```python
from build123d import *

# Parameters (mm, degrees)
SKETCH1_W           = 290
SKETCH1_H           = 154.65
BOSS_EXTRUDE1_DEPTH = 3
SKETCH2_W           = 21
SKETCH2_H           = 40.5
CUT_EXTRUDE1_DEPTH  = 165.356793669
CUT_EXTRUDE2_DEPTH  = 165.356793669
SKETCH4_W           = 24
SKETCH4_H           = 10.25
BOSS_EXTRUDE2_DEPTH = 3


with BuildPart() as part:
    # Sketch1 → Boss-Extrude1 (new body)
    with BuildSketch(Plane(origin=(0, 0, 0), x_dir=(1, 0, 0), z_dir=(0, 1, 0))):
        Rectangle(SKETCH1_W, SKETCH1_H)
    extrude(amount=BOSS_EXTRUDE1_DEPTH)

    # Sketch2 → Cut-Extrude1 (cut, through all)
    with BuildSketch(Plane(origin=(0, 3, 0), x_dir=(1, 0, 0), z_dir=(0, 1, 0))):
        with Locations((0, 57.075)):
            Rectangle(SKETCH2_W, SKETCH2_H)
    extrude(amount=-CUT_EXTRUDE1_DEPTH, mode=Mode.SUBTRACT)

    # Sketch3 → Cut-Extrude2 (cut, through all)
    with BuildSketch(Plane(origin=(0, 3, 0), x_dir=(1, 0, 0), z_dir=(0, 1, 0))):
        Polygon((-116, -73.825), (-116, -77.325), (-88.5, -77.325), (-88.5, -66.325), (-112, -66.325), (-112, -61.825), (-124, -61.825), (-124, -73.825), align=None)
    extrude(amount=-CUT_EXTRUDE2_DEPTH, mode=Mode.SUBTRACT)

    # Sketch4 → Boss-Extrude2 (add, through all)
    with BuildSketch(Plane(origin=(0, 3, 0), x_dir=(1, 0, 0), z_dir=(0, 1, 0))):
        with Locations((-133, -82.45)):
            Rectangle(SKETCH4_W, SKETCH4_H)
    extrude(amount=-BOSS_EXTRUDE2_DEPTH)


solid = part.part
```
Check sheet for the modelled part. Datum: model origin and axes. Units: mm. Coordinates: 2 decimals unless noted, no trailing zeros. Loops run counter-clockwise (first coordinate to the right, second up) from the corner with the lowest first, then second, coordinate; pieces in that order, holes last.
1) Gauge pin test, flat ends, axial feed: pin 1 (4 mm diameter, centred on x = 49, z = 11.5, fed in from -Y); pin 2 (0.9 mm diameter, centred on x = -103.5, y = 1, fed in from +Z) (3 decimals); pin 3 (1.5 mm diameter, centred on x = 62.5, y = 1, fed in from +Z) (3 decimals). Record the tip position at first contact, or that the pin passes through.
2) Material ranges on probe 1 along X at (y, z) = (1.4, 64.5); probe 2 along X at (y, z) = (2.5, -48.5); probe 3 along Z at (x, y) = (-11, 2.4) (3 decimals), recorded low to high.
3) Sectioned sample at D-D (x = 123). Record the boundary of the cut face in (y, z) (3 decimals).
4) Sectioned sample at B-B (y = 1.5). Record the boundary of the cut face in (x, z) (3 decimals).
5) Sectioned sample at C-C (x = -7). Record the boundary of the cut face in (y, z) (3 decimals), and give its area (3 significant figures).
6) Sectioned sample at A-A (z = -42). Record the boundary of the cut face in (x, y).
Check sheet entries:
1. pin 1: stops at y = 0
1. pin 2: stops at z = 66.325
1. pin 3: stops at z = 77.325
2. probe 1: x = -145 to -124, -112 to 145
2. probe 2: x = -145 to -10.5, 10.5 to 145
2. probe 3: z = -77.325 to 77.325
3. outline: (0, -77.325) - (3, -77.325) - (3, 77.325) - (0, 77.325) - close
4. outline: (-145, -77.325) - (-10.5, -77.325) - (-10.5, -36.825) - (10.5, -36.825) - (10.5, -77.325) - (145, -77.325) - (145, 77.325) - (-88.5, 77.325) - (-88.5, 66.325) - (-112, 66.325) - (-112, 61.825) - (-124, 61.825) - (-124, 73.825) - (-116, 73.825) - (-116, 77.325) - (-121, 77.325) - (-121, 87.575) - (-145, 87.575) - close
5. outline: (0, -36.825) - (3, -36.825) - (3, 77.325) - (0, 77.325) - close
5. area: 342 mm2
6. outline: (-145, 0) - (-10.5, 0) - (-10.5, 3) - (-145, 3) - close; (10.5, 0) - (145, 0) - (145, 3) - (10.5, 3) - close
